Could you check a few things on this model? Use its own coordinates, in mm. A direction names the side the tool comes from. Coordinates: 2 decimals unless noted, no trailing zeros. Loops run counter-clockwise (first coordinate to the right, second up) from the corner with the lowest first, then second, coordinate; pieces in that order, holes last. Notation, with made-up numbers: (25.5, 31.5) - (30.5, 31.5) arc R32 ccw to (30.5, 63.5) - close; hole circle Ø8 at (5, -9.75). An arc over 180 degrees is marked (long way). Put each result on its own line as item: value. Start each with the question number.
Autodesk Inventor part; units mm, degrees
ref_plane "YZ Plane" through (0, 0, 0) normal (1, 0, 0) x (0, 1, 0)
ref_plane "XZ Plane" through (0, 0, 0) normal (0, 1, 0) x (-1, 0, 0)
ref_plane "XY Plane" through (0, 0, 0) normal (0, 0, 1) x (1, 0, 0)
sketch "Sketch1" plane through (0, 0, 0) normal (0, 0, 1) x (1, 0, 0)
  line L0 (0, 0) -> (89.1946, 0) construction
  line L1 (89.1946, 0) -> (89.1946, -45.0628) construction
  line L2 (89.1946, -45.0628) -> (0, -45.0628) construction
  line L3 (0, -45.0628) -> (0, 0) construction
  line L4 (45.8, -14.477) -> (45.8, -2.9)
  line L5 (45.8, -2.9) -> (51.6, -1.25)
  line L6 (51.6, -1.25) -> (52.2, -1.62)
  line L7 (52.2, -1.62) -> (50.8, -7.72)
  line L8 (50.8, -7.72) -> (54.3, -25.9)
  line L9 (48, -27.85) -> (50, -26.55)
  line L10 (50, -26.55) -> (54.3, -25.9)
  arc A0 (38.5438, -26.3298) -> (48, -27.85) centre (44.1464, -21.65) ccw
  arc A1 (41.9, -17.327) -> (38.5438, -26.3298) centre (43.0964, -22.9) ccw
  line L11 (43.9, -16.477) -> (45.8, -14.477)
  line L12 (41.9, -17.327) -> (43.9, -16.477)
  dimension "d26" = 45.8
  dimension "d27" = 2.9
  dimension "d29" = 5.8
  dimension "d30" = 1.65
  dimension "d31" = 0.6
  dimension "d32" = 0.37
  dimension "d33" = 6.1
  dimension "d34" = 1.4
  dimension "d36" = 3.5
  dimension "d37" = 0.65
  dimension "d38" = 4.3
  dimension "d39" = 1.3
  dimension "d40" = 2
  dimension "d41" = 7.3
  dimension "d42" = 5.7
  dimension "d44" = 1.05
  dimension "d45" = 1.25
  dimension "d46" = 20
  dimension "d47" = 0.85
  dimension "d48" = 2
  dimension "d49" = 2
  dimension "d50" = 1.9
  dimension "d65" = 23
extrude "Extrusion2" add sketch "Sketch1" along normal blind 18
fillet "Fillet1" radius 2 4 edges at (54.3, -25.9, 9) (45.8, -14.477, 9) (43.9, -16.477, 9) (50.8, -7.72, 9)
sketch "Sketch3" plane through (0, 0, 18) normal (0, 0, 1) x (1, 0, 0)
  line L0 (45.8, -2.9) -> (45.8, -13.6784)
  point P0 (51.6, -1.25)
  point P1 (0, 0)
  point P2 (46.8, -22.25)
  dimension "d54" = 1
  dimension "d55" = 21
hole "Hole1" at (46.8, -22.25, 18) direction (0, 0, -1) diameter 4.5 end through all
properties part number "ExtruderSatoerCam"
(1) For pin 1 Ø5 at (y, z) = (-5, 8.5) entering from +X; pin 2 Ø5 at (y, z) = (-21, 6.5) entering from +X; pin 3 Ø2 at (x, z) = (48, 7.5) entering from +Y, each with a flat end and sliding along its axis, tell me the tip position at first contact or that it passes through.
(2) I want a section at D-D on y = -10.25. List the corners of the cut face in (x, z) for me.
(3) I want a section at B-B on x = 47.5. List the corners of the cut face in (y, z) for me.
(4) Which directions (+Z, -Z, +X, -X, +Y, -Y) give clear straight access to the entire face, cutting with the end or side of a thin tool? Please do faces 4 (the flat face through (45.8, -8, 9)), 5 (the flat face through (52.37, -15.88, 8.87)), 6 (the flat face through (51.105, -26.383, 8.874)).
(5) I need wall thicknesses on L1, parallel to Y at x = 46.8, z = 7.5; L2, parallel to X at y = -22.25, z = 6; L3, parallel to Y at x = 46.5, z = 14.25. Which ranges of each line are inside material? Lowest first, please. Write a range as [from, to].
(6) If we mould it in two halves opening along Y, with no side actions, what happens to faces 1 (the flat face through (49, -27.2, 8.9)), 2 (the flat face through (51.556, -4.425, 8.874)), 3 (the flat face through (47, -18, 18))? For each: pulls with the +Y half, pulls with the -Y half, needs draft (parallel to the pull), parting line crosses it, or undercut.
(7) I want a section at A-A on z = 2.75. List the corners of the cut face in (x, y) for me.
(8) I want a section at C-C on y = -22.25. List the corners of the cut face in (x, z) for me, and give its area (3 significant figures).
Answer sheet:
1. pin 1: stops at x = 52
1. pin 2: stops at x = 53.84
1. pin 3: stops at y = -1.99
2. outline: (45.8, 0) - (51.29, 0) - (51.29, 18) - (45.8, 18) - close
3. outline: (-28.13, 0) - (-24.39, 0) - (-24.39, 18) - (-28.13, 18) - close; (-20.11, 0) - (-2.42, 0) - (-2.42, 18) - (-20.11, 18) - close
4. face 4: +Z, -Z, -X, +Y
4. face 5: +Z, -Z, +X
4. face 6: +Z, -Z, +X, -Y
5. L1: y = [-28.45, -24.5], [-20, -2.62]
5. L2: x = [37.43, 44.55], [49.05, 53.6]
5. L3: y = [-28.56, -24.48], [-20.02, -2.7]
6. face 1: pulls with the -Y half
6. face 2: undercut
6. face 3: needs draft
7. outline: (38.54, -26.33) arc R7.3 ccw to (48, -27.85) - (50, -26.55) - (52.24, -26.21) arc R2 ccw to (53.91, -23.86) - (50.88, -8.13) arc R2 cw to (50.89, -7.31) - (52.2, -1.62) - (51.6, -1.25) - (45.8, -2.9) - (45.8, -13.68) arc R2 cw to (45.25, -15.06) - (44.19, -16.18) arc R2 cw to (43.52, -16.64) - (41.9, -17.33) arc R5.7 ccw to start; hole circle Ø4.5 at (46.8, -22.25)
8. outline: (37.43, 0) - (44.55, 0) - (44.55, 18) - (37.43, 18) - close; (49.05, 0) - (53.6, 0) - (53.6, 18) - (49.05, 18) - close
8. area: 210 mm^2
